Verification items for this drawing (mm, ordinates from the low corner). A direction names the side the tool comes from. Round coordinates to 2 decimals unless told otherwise and drop trailing zeros. Write each loop counter-clockwise with the first axis right and the second up, starting at its lowest first coordinate (ties: lowest second). Pieces come first, ordered by that corner, then holes.
Item 1: Access from +Z, -Z, +X, -X, +Y, -Y to the whole of each face (thin tool, end or side, straight path). Record for the marked faces 1 and 2.
Item 2: Cross-section at A-A (y = 37). Enter the section's corners in (x, z), then the cut area to 3 significant figures.
Item 3: Cross-section at D-D (x = 25). Enter the section's corners in (y, z).
Item 4: Scan lines: probe 1 along Y at (x, z) = (61.8, 19.45); probe 2 along Y at (x, z) = (52, 14.5); probe 3 along Z at (x, y) = (38, 21). Record each from-to range of solid material in increasing order.
Item 5: Cross-section at C-C (z = 10.5). Enter the section's corners in (x, y), then the cut area to 3 significant figures.
Item 6: Cross-section at B-B (x = 61.8). Enter the section's corners in (y, z).
Item 7: Depth check by flat-ended pin: P1, Ø14, axis at x = 31, y = 28.5, coming from the -Z side; P2, Ø7.5, axis at x = 6.2, y = 37, coming from the +Z side; P3, Ø4, axis at y = 25.5, z = 14.5, coming from the +X side. Enter the tip coordinate at first touch or a pass-through.
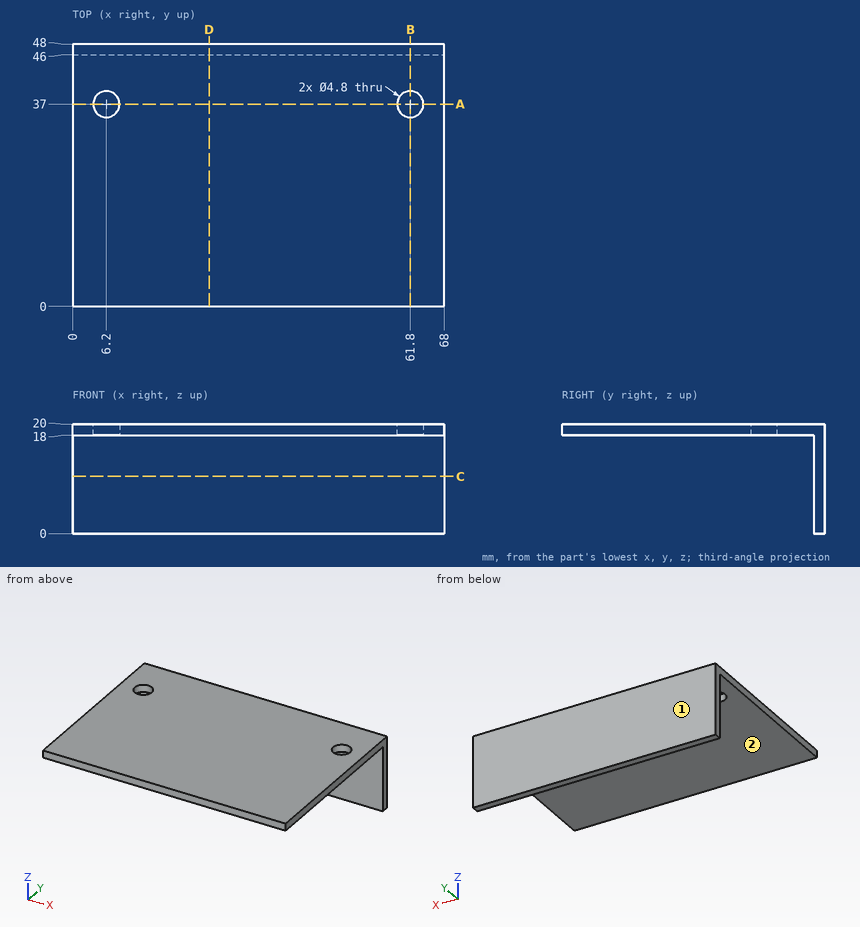
Resolved:
1. face 1: +Z, -Z, +X, -X, +Y
1. face 2: -Z, +X, -X, -Y
2. outline: (0, 18) - (3.8, 18) - (3.8, 20) - (0, 20) - close; (8.6, 18) - (59.4, 18) - (59.4, 20) - (8.6, 20) - close; (64.2, 18) - (68, 18) - (68, 20) - (64.2, 20) - close
2. area: 117 mm2
3. outline: (0, 18) - (46, 18) - (46, 0) - (48, 0) - (48, 20) - (0, 20) - close
4. probe 1: y = 0 to 34.6, 39.4 to 48
4. probe 2: y = 46 to 48
4. probe 3: z = 18 to 20
5. outline: (0, 46) - (68, 46) - (68, 48) - (0, 48) - close
5. area: 136 mm2
6. outline: (0, 18) - (34.6, 18) - (34.6, 20) - (0, 20) - close; (39.4, 18) - (46, 18) - (46, 0) - (48, 0) - (48, 20) - (39.4, 20) - close
7. P1: stops at z = 18
7. P2: stops at z = 20
7. P3: passes through
